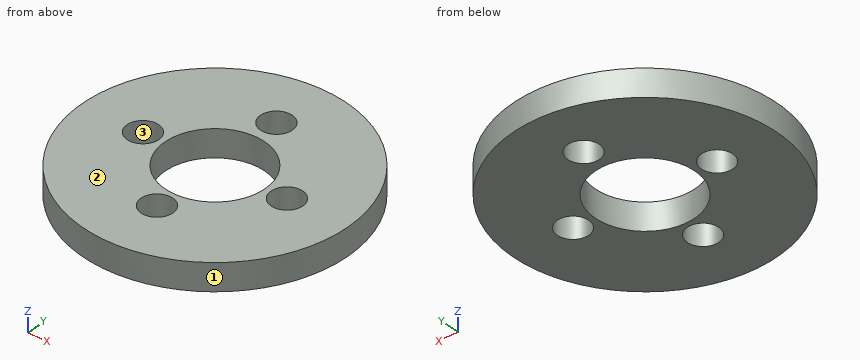
from build123d import *

# Parameters (mm, degrees)
SKETCH1_R           = 14.554642106
SKETCH1_R_2         = 1.75
BOSS_EXTRUDE1_DEPTH = 3
SKETCH2_R           = 5.5
CUT_EXTRUDE1_DEPTH  = 3


with BuildPart() as part:
    # Sketch1 → Boss-Extrude1 (new body)
    with BuildSketch(Plane.XY):
        Circle(SKETCH1_R)
        with Locations((0, 8.228052911)):
            Circle(SKETCH1_R_2, mode=Mode.SUBTRACT)
        with Locations((-7.85825278, 0)):
            Circle(SKETCH1_R_2, mode=Mode.SUBTRACT)
        with Locations((0, -7.765802747)):
            Circle(SKETCH1_R_2, mode=Mode.SUBTRACT)
        with Locations((7.85825278, 0)):
            Circle(SKETCH1_R_2, mode=Mode.SUBTRACT)
    extrude(amount=BOSS_EXTRUDE1_DEPTH)

    # Sketch2 → Cut-Extrude1 (cut)
    with BuildSketch(Plane.XY.offset(3)):
        Circle(SKETCH2_R)
    extrude(amount=-CUT_EXTRUDE1_DEPTH, mode=Mode.SUBTRACT)


solid = part.part
The model under review builds one solid part; all positions refer to its coordinate system, in mm. Face numbers are marked on the shaded views. Round coordinates to 2 decimals unless told otherwise and drop trailing zeros. Write each loop counter-clockwise with the first axis right and the second up, starting at its lowest first coordinate (ties: lowest second). Pieces come first, ordered by that corner, then holes. Notation, with made-up numbers: M 4,-15.5 L 31,-15.5 A27 ccw 31,8.5 Z; hole C 1.5,53 d7. An arc over 180 degrees is marked long. Answer as CSV lines item,"result". Start each with the question number.
Q1. Wall thickness on line 1 along Y through (x, z) = (0, 1.6); line 2 along Y through (x, z) = (-1.5, 2.55); line 3 along X through (y, z) = (0.75, 2.3): over which ranges is each line inside the solid? List them lowest first.
Q2. Consider section C-C, the plane y = 8.75. Give the boundary of the cut face in (x, z).
Q3. Consider section B-B, the plane x = 0. Give the boundary of the cut face in (y, z), then the cut area to 3 significant figures.
Q4. The part is to be moulded in two halves that separate along X. For the marked faces 1, 2 and 3, say which applies: +X half, -X half, draft (parallel to the pull), parting line (faces both ways), or undercut.
Q5. Consider section A-A, the plane y = 0. Give the boundary of the cut face in (x, z).
Q6. Consider section D-D, the plane z = 0.7. Give the boundary of the cut face in (x, y).
Q7. Clearance check with a flat-ended pin moving along its axis: P1, Ø1.5, axis at x = -5.5, z = 0.5, coming from the -Y side. State where the tip first meets the part, or that it passes through.
Result set:
1,line 1,"y = -14.55 to -9.52, -6.02 to -5.5, 5.5 to 6.48, 9.98 to 14.55"
1,line 2,"y = -14.48 to -8.67, -6.86 to -5.29, 5.29 to 7.33, 9.13 to 14.48"
1,line 3,"x = -14.54 to -9.44, -6.28 to -5.45, 5.45 to 6.28, 9.44 to 14.54"
2,outline,"M -11.63,0 L -1.67,0 L -1.67,3 L -11.63,3 Z; M 1.67,0 L 11.63,0 L 11.63,3 L 1.67,3 Z"
3,outline,"M -14.55,0 L -9.52,0 L -9.52,3 L -14.55,3 Z; M -6.02,0 L -5.5,0 L -5.5,3 L -6.02,3 Z; M 5.5,0 L 6.48,0 L 6.48,3 L 5.5,3 Z; M 9.98,0 L 14.55,0 L 14.55,3 L 9.98,3 Z"
3,area,"33.3 mm²"
4,face 1,"parting line"
4,face 2,"draft"
4,face 3,"undercut"
5,outline,"M -14.55,0 L -9.61,0 L -9.61,3 L -14.55,3 Z; M -6.11,0 L -5.5,0 L -5.5,3 L -6.11,3 Z; M 5.5,0 L 6.11,0 L 6.11,3 L 5.5,3 Z; M 9.61,0 L 14.55,0 L 14.55,3 L 9.61,3 Z"
6,outline,"C 0,0 d29.11; hole C -7.86,0 d3.5; hole C 0,0 d11; hole C 0,-7.77 d3.5; hole C 0,8.23 d3.5; hole C 7.86,0 d3.5"
7,P1,"stops at y = -13.76"
